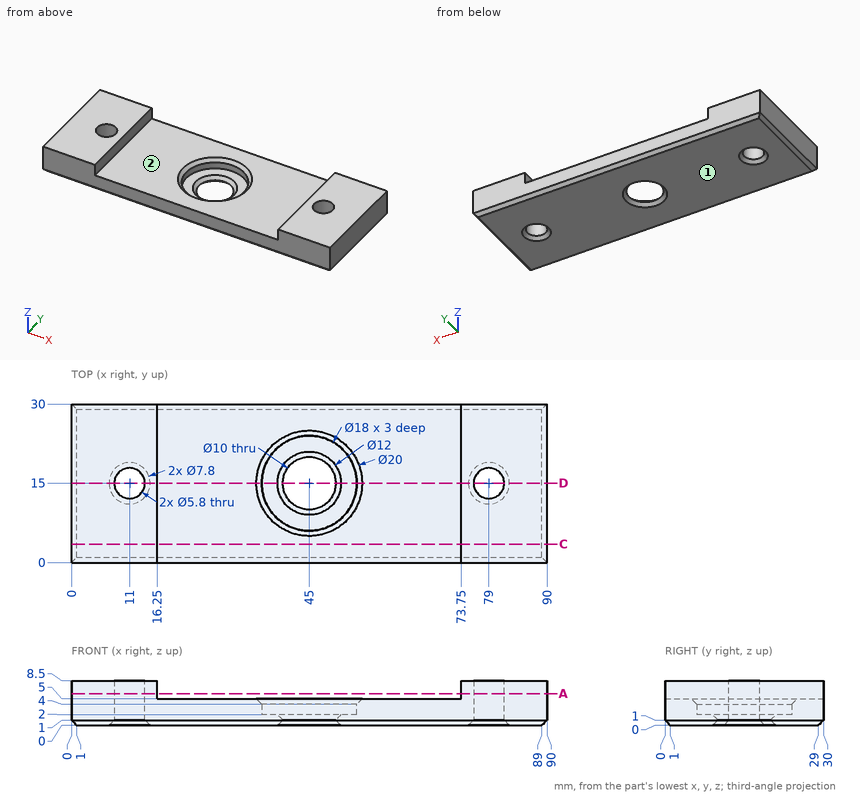
Can you work these out from the drawing? Everything is in mm from the part's minimum corner. Round coordinates to 2 decimals unless told otherwise and drop trailing zeros. Loops run counter-clockwise (first coordinate to the right, second up) from the corner with the lowest first, then second, coordinate; pieces in that order, holes last. Notation, with made-up numbers: (64, 21.5) -> (81, 21.5) arc R11 cw to (81, 31.5) -> close; hole circle Ø11 at (24, 22). An arc over 180 degrees is marked (long way). Answer in a Markdown table with one row per item.
Item 1: Suppose I cut it at C-C, the plane y = 3.5. List the corners of the cut face in (x, z) for me, plus the area to 3 significant figures.
Answer block:
| item | result |
|---|---|
| outline | (0, 1) -> (1, 0) -> (89, 0) -> (90, 1) -> (90, 8.5) -> (73.75, 8.5) -> (73.75, 5) -> (16.25, 5) -> (16.25, 8.5) -> (0, 8.5) -> close |
| area | 563 mm² |
Item 2: Will these pins go through, and if not, where does the flat tip stop? P1, Ø9, axis at x = 36.5, y = 15.5, coming from the +Z side; P2, Ø4.5, axis at x = 11, y = 15, coming from the +Z side; P3, Ø6, axis at x = 73.5, y = 4.5, coming from the +Z side.
Answer block:
| item | result |
|---|---|
| P1 | z = 5 |
| P2 | through |
| P3 | z = 8.5 |
Item 3: If I drill on probe 1 along Y at (x, z) = (79, 5.5); probe 2 along X at (y, z) = (17.5, 1.25) (1 decimal); probe 3 along Z at (x, y) = (59, 14), over which ranges is the centre line in solid material (lowest first)?
Answer block:
| item | result |
|---|---|
| probe 1 | 0 to 12.1, 17.9 to 30 |
| probe 2 | 0 to 9.5, 12.5 to 40.4, 49.6 to 77.5, 80.5 to 90 |
| probe 3 | 0 to 5 |
Item 4: Suppose I cut it at A-A, the plane z = 6. List the corners of the cut face in (x, y) for me.
Answer block:
| item | result |
|---|---|
| outline | (0, 0) -> (16.25, 0) -> (16.25, 30) -> (0, 30) -> close; (73.75, 0) -> (90, 0) -> (90, 30) -> (73.75, 30) -> close; hole circle Ø5.8 at (11, 15); hole circle Ø5.8 at (79, 15) |
Item 5: Suppose I cut it at D-D, the plane y = 15. Give the number of separate pieces and of enclosed holes in the cut face, plus the area to 3 significant figures.
Answer block:
| item | result |
|---|---|
| separate pieces | 4 |
| enclosed holes | 0 |
| area | 385 mm² |
Item 6: We'd pull the mould along X, two halves only. Please class the marked faces 1 and 2: released by +X, released by -X, zero draft, split by the parting line, or undercut.
Answer block:
| item | result |
|---|---|
| face 1 | zero draft |
| face 2 | undercut |
